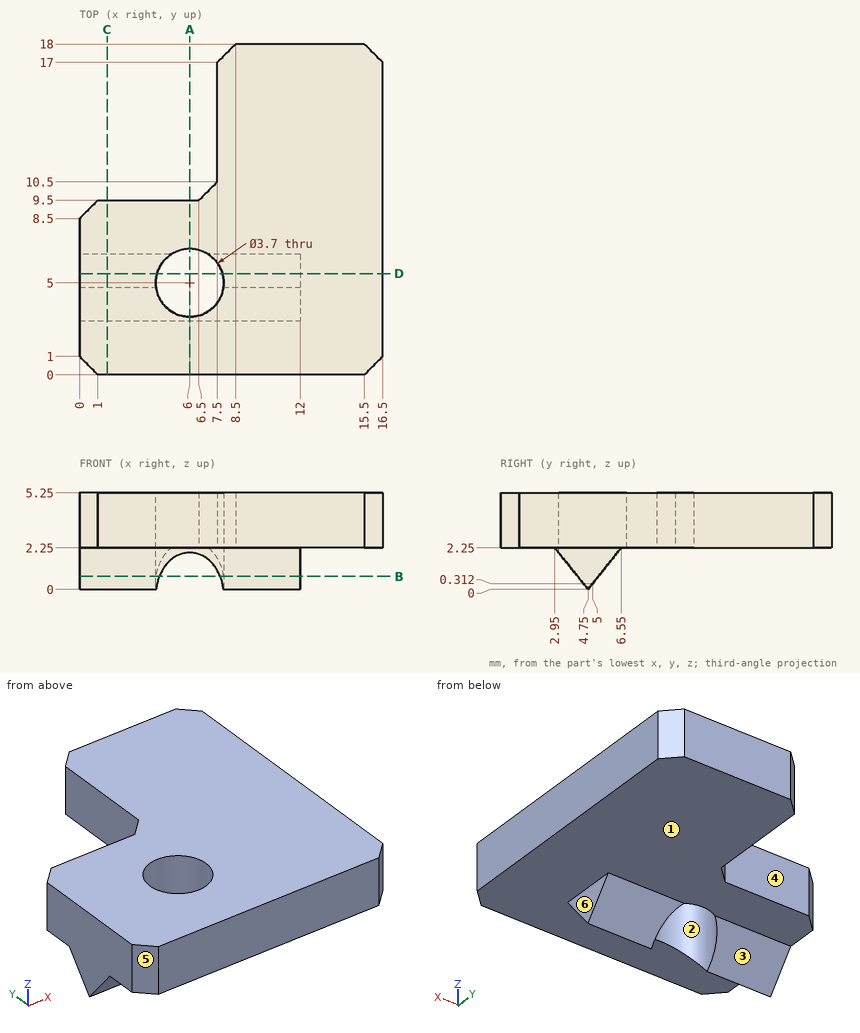
Here's the drawing with two shaded views (mm, measured from the low corner). I have some questions. A direction names the side the tool comes from. Give positions to 0.01 mm unless a question says otherwise; leave off trailing zeros. Order: outer loops, then holes, each group sorted by start corner. A loop starts at its lowest first (then second) coordinate and runs counter-clockwise, first axis right, second up.
Q1. I'm going to push flat-ended pins straight in: P1, Ø1.5, axis at x = 4.5, z = 3.5, coming from the +Y side; P2, Ø0.9, axis at y = 13, z = 3, coming from the -X side. Where does each tip first touch, or does it pass through?
Q2. We'd pull the mould along Y, two halves only. Please class the marked faces 1, 2 and 3: +Y half, -Y half, draft (parallel to the pull), parting line (faces both ways), or undercut.
Q3. Suppose I cut it at B-B, the plane z = 0.7. Write out the boundary of the cut face in (x, y).
Q4. If I drill on line 1 along Y through (x, z) = (6, 4.05); line 2 along X through (y, z) = (5, 4.1); line 3 along X through (y, z) = (5, 1.2), over which ranges is the centre line in solid material (lowest first)?
Q5. For the marked faces 4, 5 and 6, which set-ups out of +Z, -Z, +X, -X, +Y, -Y let a thin tool reach every point of the face, with its end or its side?
Q6. Suppose I cut it at C-C, the plane x = 1.5. Write out the boundary of the cut face in (y, z).
Q7. Suppose I cut it at D-D, the plane y = 5.5. Write out the boundary of the cut face in (x, z).
Q8. Suppose I cut it at A-A, the plane x = 6. Write out the boundary of the cut face in (y, z).
Solution:
1. P1: stops at y = 9.5
1. P2: stops at x = 7.5
2. face 1: draft
2. face 2: undercut
2. face 3: +Y half
3. outline: (0, 4.19) - (4.34, 4.19) arc R1.85 cw to (4.18, 5.31) - (0, 5.31) - close; (7.66, 4.19) - (12, 4.19) - (12, 5.31) - (7.82, 5.31) arc R1.85 cw to start
4. line 1: y = 0 to 3.15, 6.85 to 9.5
4. line 2: x = 0 to 4.15, 7.85 to 16.5
4. line 3: x = 0 to 4.15, 7.85 to 12
5. face 4: +Z, -Z, -X, +Y
5. face 5: +Z, -Z, -X, -Y
5. face 6: -Z, +X, +Y, -Y
6. outline: (0, 2.25) - (2.95, 2.25) - (4.75, 0) - (6.55, 2.25) - (9.5, 2.25) - (9.5, 5.25) - (0, 5.25) - close
7. outline: (0, 0.94) - (4.22, 0.94) - (4.22, 5.25) - (0, 5.25) - close; (7.78, 0.94) - (12, 0.94) - (12, 2.25) - (16.5, 2.25) - (16.5, 5.25) - (7.78, 5.25) - close
8. outline: (0, 2.25) - (2.95, 2.25) - (3.15, 2) - (3.15, 5.25) - (0, 5.25) - close; (6.85, 2.25) - (9.5, 2.25) - (9.5, 5.25) - (6.85, 5.25) - close
